Here's how the part is built. I have some questions about the finished solid (model axes, mm). A direction names the side the tool comes from. Give positions to 0.01 mm unless a question says otherwise; leave off trailing zeros. Loops run counter-clockwise (first coordinate to the right, second up) from the corner with the lowest first, then second, coordinate; pieces in that order, holes last. Notation, with made-up numbers: (78, 71.5) -> (115, 71.5) arc R19 ccw to (115, 106.5) -> close; hole circle Ø4 at (17.25, -14.75). An arc over 180 degrees is marked (long way). Answer in a Markdown table with one row per item. Add a question column.
Item 1: Which directions (+Z, -Z, +X, -X, +Y, -Y) give clear straight access to the entire face, cutting with the end or side of a thin tool? Please do faces 5 (the face through (-0.54, -2.44, 2.71)), 6 (the face through (8.554, -0.23, 0.838)), 7 (the face through (1, 1, 1)).
Item 2: For P1, Ø1.6, axis at x = 10, y = 0, coming from the +Z side; P2, Ø1, axis at y = -2.5, z = 3, coming from the +X side; P3, Ø1.9, axis at x = 12, y = 0, coming from the -Z side; P4, Ø3, axis at x = 0, y = 0, coming from the -Z side, each with a flat end and sliding along its axis, tell me the tip position at first contact or that it passes through.
Item 3: If we section it at D-D (y = 1.5): Write out the boundary of the cut face in (x, z).
Item 4: If we section it at A-A (z = 0.45): Give the number of separate pieces and of enclosed holes in the cut face, then the cut area to 3 significant figures.
Item 5: If we section it at B-B (x = 4): Write out the boundary of the cut face in (y, z), then the cut area to 3 significant figures.
Item 6: We'd pull the mould along Y, two halves only. Please class faces 1 (the face through (0, -3, 0)), 2 (the face through (-15.916, 0.043, 0.838)), 3 (the face through (11.4, 0, 0.8)), 4 (the face through (-0.54, 2.44, 0.49)): released by +Y, released by -Y, zero draft, split by the parting line, or undercut.
Item 7: If I drill on line 1 (Y direction, x = 0, z = 0.3); line 2 (Y direction, x = -14, z = 0.6); line 3 (Z direction, x = 8.5, y = -0.5), over which ranges is the centre line in solid material (lowest first)?
```python
from build123d import *

# Parameters (mm, degrees)
F0_R     = 0.6
F1_DEPTH = 1.7
F2_R     = 3.35
F3_DEPTH = 2
F4_R     = 2.5
F5_DEPTH = 1
F6_R     = 1.1
F7_DEPTH = 2.701
F8_R     = 2.5
F9_DEPTH = 2


with BuildPart() as f1:
    # F0 (on Top) → F1 (new body)
    with BuildSketch(Plane.XY):
        with BuildLine():
            ThreePointArc((2.2299103121, -2.5), (3.057180036, -1.369726333), (3.35, 0))
            ThreePointArc((3.35, 0), (3.057180036, 1.369726333), (2.2299103121, 2.5))
            ThreePointArc((2.2299103121, 2.5), (0, 3.35), (-2.2299103121, 2.5))
            ThreePointArc((-2.2299103121, 2.5), (-3.35, 0), (-2.2299103121, -2.5))
            ThreePointArc((-2.2299103121, -2.5), (0, -3.35), (2.2299103121, -2.5))
        make_face()
        with BuildLine():
            ThreePointArc((2.2299103121, 2.5), (3.057180036, 1.369726333), (3.35, 0))
            ThreePointArc((3.35, 0), (3.057180036, -1.369726333), (2.2299103121, -2.5))
            Line((2.2299103121, -2.5), (14, -2))
            ThreePointArc((14, -2), (15.9168426648, 0), (14, 2))
            Line((14, 2), (2.2299103121, 2.5))
        make_face()
        with Locations((4, 0)):
            Circle(F0_R, mode=Mode.SUBTRACT)
        with Locations((6, 0)):
            Circle(F0_R, mode=Mode.SUBTRACT)
        with Locations((8, 0)):
            Circle(F0_R, mode=Mode.SUBTRACT)
        with Locations((10, 0)):
            Circle(F0_R, mode=Mode.SUBTRACT)
        with Locations((12, 0)):
            Circle(F0_R, mode=Mode.SUBTRACT)
        with Locations((14, 0)):
            Circle(F0_R, mode=Mode.SUBTRACT)
        with BuildLine():
            ThreePointArc((-2.2299103121, -2.5), (-3.35, 0), (-2.2299103121, 2.5))
            Line((-2.2299103121, 2.5), (-14, 2))
            ThreePointArc((-14, 2), (-15.9168426648, 0), (-14, -2))
            Line((-14, -2), (-2.2299103121, -2.5))
        make_face()
        with Locations((-14, 0)):
            Circle(F0_R, mode=Mode.SUBTRACT)
        with Locations((-12, 0)):
            Circle(F0_R, mode=Mode.SUBTRACT)
        with Locations((-10, 0)):
            Circle(F0_R, mode=Mode.SUBTRACT)
        with Locations((-8, 0)):
            Circle(F0_R, mode=Mode.SUBTRACT)
        with Locations((-6, 0)):
            Circle(F0_R, mode=Mode.SUBTRACT)
        with Locations((-4, 0)):
            Circle(F0_R, mode=Mode.SUBTRACT)
    extrude(amount=F1_DEPTH)

    # F2 (on face) → F3 (join)
    with BuildSketch(Plane.XY.offset(1.7)):
        Circle(F2_R)
    extrude(amount=F3_DEPTH)

    # F4 (on face) → F5 (cut)
    with BuildSketch(Plane(origin=(0, 0, 0), x_dir=(1, 0, 0), z_dir=(0, 0, -1))):
        Circle(F4_R)
    extrude(amount=-F5_DEPTH, mode=Mode.SUBTRACT)

    # F6 (on face) → F7 (cut, through all)
    with BuildSketch(Plane(origin=(0, 0, 1), x_dir=(1, 0, 0), z_dir=(0, 0, -1))):
        Circle(F6_R)
    extrude(amount=-F7_DEPTH, mode=Mode.SUBTRACT)

    # F8 (on face) → F9 (cut)
    with BuildSketch(Plane.XY.offset(3.7)):
        Circle(F8_R)
    extrude(amount=-F9_DEPTH, mode=Mode.SUBTRACT)


solid = f1.part
```
Recorded:
| question | item | result |
|---|---|---|
| 1 | face 5 | +Z |
| 1 | face 6 | +Z, -Z |
| 1 | face 7 | -Z |
| 2 | P1 | stops at z = 1.7 |
| 2 | P2 | stops at x = 2.69 |
| 2 | P3 | stops at z = 0 |
| 2 | P4 | stops at z = 1 |
| 3 | outline | (-15.24, 0) -> (-2, 0) -> (-2, 1) -> (2, 1) -> (2, 0) -> (15.24, 0) -> (15.24, 1.7) -> (3, 1.7) -> (3, 3.7) -> (2, 3.7) -> (2, 1.7) -> (-2, 1.7) -> (-2, 3.7) -> (-3, 3.7) -> (-3, 1.7) -> (-15.24, 1.7) -> close |
| 4 | separate pieces | 1 |
| 4 | enclosed holes | 13 |
| 4 | area | 112 mm^2 |
| 5 | outline | (-2.42, 0) -> (-0.6, 0) -> (-0.6, 1.7) -> (-2.42, 1.7) -> close; (0.6, 0) -> (2.42, 0) -> (2.42, 1.7) -> (0.6, 1.7) -> close |
| 5 | area | 6.20 mm^2 |
| 6 | face 1 | zero draft |
| 6 | face 2 | split by the parting line |
| 6 | face 3 | undercut |
| 6 | face 4 | undercut |
| 7 | line 1 | y = -3.35 to -2.5, 2.5 to 3.35 |
| 7 | line 2 | y = -2 to -0.6, 0.6 to 2 |
| 7 | line 3 | z = 0 to 1.7 |
